Geometry: final body of the model. Coordinates: model frame, mm. A direction names the side the tool comes from. Coordinates: 2 decimals unless noted, no trailing zeros. Order: outer loops, then holes, each group sorted by start corner. A loop starts at its lowest first (then second) coordinate and runs counter-clockwise, first axis right, second up. Notation, with made-up numbers: M 46,71 L 64,71 A31 cw 64,95 Z; hole C 56,-21 d6. An arc over 180 degrees is marked long. Write item = value, one per line. Start each with the question number.
```python
from build123d import *

# Parameters (mm, degrees)
F1_DEPTH = 12.7


with BuildPart() as f1:
    # F0 (on Front) → F1 (new body)
    with BuildSketch(Plane.XZ):
        Polygon((-29.21, 0), (0, 0), (0, 8.128), (-6.604, 8.128), (-6.604, 4.318), (-7.62, 4.318), (-7.62, 9.906), (-29.21, 9.906), align=None)
    extrude(amount=F1_DEPTH)

    # F2: F1 across face


with BuildPart() as f1_1:
    add(f1.part)
    add(f1.part.mirror(Plane(origin=(-14.605, -6.35, 0), x_dir=(1, 0, 0), z_dir=(0, 0, -1))))

    # F3: F1 across face


with BuildPart() as f1_2:
    add(f1_1.part)
    add(f1_1.part.mirror(Plane(origin=(0, -6.35, 0), x_dir=(0, 1, 0), z_dir=(1, 0, 0))))


solid = f1_2.part
```
Item 1: Material intervals for probe 1 along X at (y, z) = (-8.25, -7); probe 2 along X at (y, z) = (-5.5, -8.5); probe 3 along Z at (x, y) = (7.5, -6.75), sorted ascending. Write a range as [from, to].
Item 2: Draft query along X for faces 4 (the flat face through (-7.62, -6, 7)), 5 (the flat face through (-29.21, -6, 0)), 6 (the flat face through (0, 0, 0)). Return one class per face: pulls with the +X half, pulls with the -X half, needs draft (parallel to the pull), parting line crosses it, or undercut.
Item 3: Section query A-A on y = -4.5. Output: boundary loops of the cut face in (x, z).
Item 4: Reachability of faces 1 (the flat face through (6.604, -6, 6)), 2 (the flat face through (-7, -6, -4.318)), 3 (the flat face through (-18, -6, 9.906)) from +Z, -Z, +X, -X, +Y, -Y: full face, straight path, thin tool, end or side. Return the list, or none.
Item 5: First-contact query: pin 1 (1.1 mm diameter, centred on x = -7, y = -4, fed in from -Z). Flat tip, straight axial feed; report the tip coordinate or a pass-through.
Item 6: Section query B-B on z = -6.25. Output: boundary loops of the cut face in (x, y), and give its area (3 significant figures).
Item 7: Section query C-C on x = 6. Output: boundary loops of the cut face in (y, z), and give its area (3 significant figures).
Ans:
q1.probe_1 = [-29.21, -7.62], [-6.6, 6.6], [7.62, 29.21]
q1.probe_2 = [-29.21, -7.62], [7.62, 29.21]
q1.probe_3 = [-4.32, 4.32]
q2.face_4 = undercut
q2.face_5 = pulls with the -X half
q2.face_6 = needs draft
q3.outline = M -29.21,-9.91 L -7.62,-9.91 L -7.62,-4.32 L -6.6,-4.32 L -6.6,-8.13 L 6.6,-8.13 L 6.6,-4.32 L 7.62,-4.32 L 7.62,-9.91 L 29.21,-9.91 L 29.21,9.91 L 7.62,9.91 L 7.62,4.32 L 6.6,4.32 L 6.6,8.13 L -6.6,8.13 L -6.6,4.32 L -7.62,4.32 L -7.62,9.91 L -29.21,9.91 Z
q4.face_1 = +Z, +Y, -Y
q4.face_2 = -Z, +Y, -Y
q4.face_3 = +Z, +X, -X, +Y, -Y
q5.pin_1 = -8.13
q6.outline = M -29.21,-12.7 L -7.62,-12.7 L -7.62,0 L -29.21,0 Z; M -6.6,-12.7 L 6.6,-12.7 L 6.6,0 L -6.6,0 Z; M 7.62,-12.7 L 29.21,-12.7 L 29.21,0 L 7.62,0 Z
q6.area = 716 mm^2
q7.outline = M -12.7,-8.13 L 0,-8.13 L 0,8.13 L -12.7,8.13 Z
q7.area = 206 mm^2
